```python
from build123d import *

# Parameters (mm, degrees)
F0_W      = 62.4516925456
F0_H      = 19.2159049461
F1_DEPTH  = 2.54
F0_W_2    = 5.240462238
F0_H_2    = 12.7
F1_FACE_W = 62.4516925456
F1_FACE_H = 19.2159049461
F2_DEPTH  = 2.54
F3_DEPTH  = 2.54
F4_DEPTH  = 12.7
F5_W      = 9.6827298403
F5_H      = 24.7204606325
F5_W_2    = 9.949860665
F6_DEPTH  = 35.56
F7_W      = 6.4173687831
F7_H      = 20.8289548615
F8_DEPTH  = 10.16
F9_W      = 6.6844996078
F9_H      = 20.8289548615
F10_DEPTH = 10.16
F11_W     = 6.4173687831
F11_H     = 20.8289548615
F12_DEPTH = 7.62
F13_W     = 6.6844996078
F13_H     = 20.8289548615
F14_DEPTH = 7.62
F16_D     = 1.27
F16_DEPTH = 127
F16_TIP   = 0.3815464931
F17_W     = 5.240462238
F17_H     = 12.7
F18_DEPTH = 39.37


with BuildPart() as f1:
    # F0 (on Top) → F1 (new body)
    with BuildSketch(Plane.XY):
        with Locations((34.3284141645, -12.7105206001)):
            Rectangle(F0_W, F0_H)
    extrude(amount=F1_DEPTH)

    # F0 (on Top) + F1_face (on face) → F2 (join)
    with BuildSketch(Plane.XY):
        Polygon((71.280462238, 0), (0, 0), (0, -24.7204606325), (33.02, -24.7204606325), (38.260462238, -24.7204606325), (71.280462238, -24.7204606325), align=None)
        with Locations((34.3284141645, -12.7105206001)):
            Rectangle(F0_W, F0_H, mode=Mode.SUBTRACT)
        with Locations((35.640231119, -31.0704606325)):
            Rectangle(F0_W_2, F0_H_2)
    with BuildSketch(Plane(origin=(34.3284141645, -12.7105206001, 0), x_dir=(1, 0, 0), z_dir=(0, 0, -1))):
        Rectangle(F1_FACE_W, F1_FACE_H)
    extrude(amount=F2_DEPTH, dir=(0, 0, 1))

    # F0 (on Top) → F3 (join)
    with BuildSketch(Plane.XY):
        with Locations((34.3284141645, -12.7105206001)):
            Rectangle(F0_W, F0_H)
    extrude(amount=-F3_DEPTH)

    # F0 (on Top) → F4 (join)
    with BuildSketch(Plane.XY):
        with Locations((35.640231119, -31.0704606325)):
            Rectangle(F0_W_2, F0_H_2)
    extrude(amount=F4_DEPTH)

    # F5 (on face) → F6 (join)
    with BuildSketch(Plane.XY.offset(2.54)):
        with Locations((4.8413649201, -12.3602303163)):
            Rectangle(F5_W, F5_H)
        with Locations((66.3055319055, -12.3602303163)):
            Rectangle(F5_W_2, F5_H)
    extrude(amount=F6_DEPTH)

    # F7 (on face) → F8 (join)
    with BuildSketch(Plane.XY.offset(38.1)):
        with Locations((4.8413649201, -12.3602303163)):
            Rectangle(F7_W, F7_H)
    extrude(amount=F8_DEPTH)

    # F9 (on face) → F10 (join)
    with BuildSketch(Plane.XY.offset(38.1)):
        with Locations((66.3055319055, -12.3602303163)):
            Rectangle(F9_W, F9_H)
    extrude(amount=F10_DEPTH)

    # F11 (on face) → F12 (join)
    with BuildSketch(Plane.XY.offset(48.26)):
        Polygon((8.7310628216, -1.3743147005), (0.9516670187, -1.3743147005), (1.6326805286, -1.9457528855), (8.0500493117, -1.9457528855), (8.0500493117, -22.774707747), (8.7310628216, -23.346145932), align=None)
        Polygon((1.6326805286, -1.9457528855), (0.9516670187, -1.3743147005), (0.9516670187, -23.346145932), (8.7310628216, -23.346145932), (8.0500493117, -22.774707747), (1.6326805286, -22.774707747), align=None)
        with Locations((4.8413649201, -12.3602303163)):
            Rectangle(F11_W, F11_H)
    extrude(amount=F12_DEPTH)

    # F13 (on face) → F14 (join)
    with BuildSketch(Plane.XY.offset(48.26)):
        Polygon((70.3287952193, -1.2647393756), (62.3918439166, -1.2647393756), (62.9632821016, -1.9457528855), (69.6477817094, -1.9457528855), (69.6477817094, -22.774707747), (70.3287952193, -23.346145932), align=None)
        Polygon((62.9632821016, -1.9457528855), (62.3918439166, -1.2647393756), (62.3918439166, -23.346145932), (70.3287952193, -23.346145932), (69.6477817094, -22.774707747), (62.9632821016, -22.774707747), align=None)
        with Locations((66.3055319055, -12.3602303163)):
            Rectangle(F13_W, F13_H)
    extrude(amount=F14_DEPTH)

    # F16
    with Locations(Plane(origin=(0.9516670187, 0, 0), x_dir=(0, -1, 0), z_dir=(-1, 0, 0))):
        with Locations((5.6923147005, 52.07)):
            Hole(F16_D / 2, depth=F16_DEPTH)
            with Locations((0, 0, -(F16_DEPTH + F16_TIP / 2))):  # 118° drill point
                Cone(0, F16_D / 2, F16_TIP, mode=Mode.SUBTRACT)

    # F17 (on face) → F18 (join)
    with BuildSketch(Plane.XY.offset(12.7)):
        Polygon((40.2326633617, -17.3601058362), (31.0477988763, -17.3601058362), (33.02, -24.7204606325), (38.260462238, -24.7204606325), (38.260462238, -37.4204606325), (40.2326633617, -44.7808154288), align=None)
        Polygon((33.02, -24.7204606325), (31.0477988763, -17.3601058362), (31.0477988763, -44.7808154288), (40.2326633617, -44.7808154288), (38.260462238, -37.4204606325), (33.02, -37.4204606325), align=None)
        with Locations((35.640231119, -31.0704606325)):
            Rectangle(F17_W, F17_H)
    extrude(amount=F18_DEPTH)


solid = f1.part
```
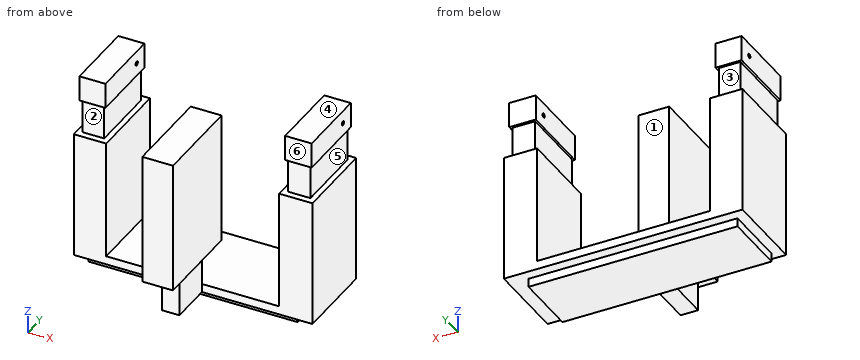
Check sheet for the modelled part. Datum: model origin and axes. Units: mm. Face numbers are marked on the shaded views. A direction names the side the tool comes from. Round coordinates to 2 decimals unless told otherwise and drop trailing zeros. Loops run counter-clockwise (first coordinate to the right, second up) from the corner with the lowest first, then second, coordinate; pieces in that order, holes last. Notation, with made-up numbers: (55, 78) - (112, 78) arc R18 cw to (112, 83) - close; hole circle Ø10 at (-6.5, 17.5). An arc over 180 degrees is marked (long way). Answer as a JSON object with one key per item and string values. Group by question number.
Q1. Mould release check, pull along Z, two halves, no side actions. Record for the marked faces 4, 5 and 6: released by +Z, released by -Z, zero draft, split by the parting line, or undercut.
Q2. Sectioned sample at C-C, the plane x = 64.5. Enter the section's corners in (y, z) (3 decimals).
Q3. Set-up check for the marked faces 1, 2 and 3: record each of +Z, -Z, +X, -X, +Y, -Y from which the full face is reachable in a straight line by a thin tool's end or side.
Q4. Gauge pin test, flat ends, axial feed: P1, Ø3, axis at y = -33.5, z = 4.5, coming from the -X side; P2, Ø0.8, axis at y = -11, z = -1, coming from the +X side; P3, Ø7.5, axis at x = 65.5, z = 44, coming from the +Y side. Record the tip position at first contact, or that the pin passes through.
Q5. Scan lines: line 1 along X through (y, z) = (-24.5, 17.5); line 2 along Y through (x, z) = (6, 52); line 3 along X through (y, z) = (-15, 18.5). Record each from-to range of solid material in increasing order. Write a range as [from, to].
Q6. Sectioned sample at B-B, the plane z = 32. Enter the section's corners in (x, y), plus the area to 3 significant figures.
Q7. Sectioned sample at D-D, the plane x = 29. Enter the section's corners in (y, z).
Solution:
{
 "1": {"face 4": "released by +Z", "face 5": "undercut", "face 6": "zero draft"},
 "2": {"outline": "(-24.72, 0) - (-22.318, 0) - (-22.318, -2.54) - (-3.103, -2.54) - (-3.103, 0) - (0, 0) - (0, 38.1) - (-1.946, 38.1) - (-1.946, 48.26) - (-1.265, 48.26) - (-1.265, 55.88) - (-23.346, 55.88) - (-23.346, 48.26) - (-22.775, 48.26) - (-22.775, 38.1) - (-24.72, 38.1) - close; hole circle Ø1.27 at (-5.692, 52.07)"},
 "3": {"face 1": "+Z, +Y", "face 2": "-X, -Y", "face 3": "+X, -X, +Y"},
 "4": {"P1": "stops at x = 33.02", "P2": "stops at x = 65.55", "P3": "stops at y = -1.95"},
 "5": {"line 1": "x = [0, 9.68], [31.05, 40.23], [61.33, 71.28]", "line 2": "y = [-23.35, -6.32], [-5.06, -1.37]", "line 3": "x = [0, 9.68], [61.33, 71.28]"},
 "6": {"outline": "(0, -24.72) - (9.68, -24.72) - (9.68, 0) - (0, 0) - close; (31.05, -44.78) - (40.23, -44.78) - (40.23, -17.36) - (31.05, -17.36) - close; (61.33, -24.72) - (71.28, -24.72) - (71.28, 0) - (61.33, 0) - close", "area": "737 mm²"},
 "7": {"outline": "(-24.72, 0) - (-22.32, 0) - (-22.32, -2.54) - (-3.1, -2.54) - (-3.1, 0) - (0, 0) - (0, 2.54) - (-24.72, 2.54) - close"}
}
